Design review of the part built by this model. Coordinates are the model's own, in mm. A direction names the side the tool comes from. Coordinates: 2 decimals unless noted, no trailing zeros. Loops run counter-clockwise (first coordinate to the right, second up) from the corner with the lowest first, then second, coordinate; pieces in that order, holes last. Notation, with made-up numbers: M 21,36.25 L 67,36.25 A26 ccw 67,72.25 Z; hole C -4.5,45.25 d10. An arc over 180 degrees is marked long. One line per item, written item: value.
```python
from build123d import *

# Parameters (mm, degrees)
SKETCH1_R           = 5
BOSS_EXTRUDE1_DEPTH = 45
CHAMFER1_SIZE       = 1
CUT_EXTRUDE1_START  = -2
SKETCH2_R           = 6
SKETCH2_R_2         = 4
CUT_EXTRUDE1_DEPTH  = 1
CUT_EXTRUDE2_START  = -42
SKETCH2_2_R         = 6
SKETCH2_2_R_2       = 4
CUT_EXTRUDE2_DEPTH  = 1


with BuildPart() as part:
    # Sketch1 → Boss-Extrude1 (new body)
    with BuildSketch(Plane(origin=(0, 0, 0), x_dir=(1, 0, 0), z_dir=(0, 1, 0))):
        with Locations(Location((0, 0, 0), (0, 0, 90))):
            Circle(SKETCH1_R)
    extrude(amount=BOSS_EXTRUDE1_DEPTH)

    # Chamfer1
    chamfer1_edges = [part.edges().sort_by_distance(p)[0] for p in [
        (0, 0, 5),
        (0, 45, 5),
    ]]
    chamfer(chamfer1_edges, length=CHAMFER1_SIZE)

    # Sketch2 → Cut-Extrude1 (cut)
    with BuildSketch(Plane.XZ.offset(CUT_EXTRUDE1_START)):
        Circle(SKETCH2_R)
        with Locations(Location((0, 0, 0), (0, 0, 270))):
            Circle(SKETCH2_R_2, mode=Mode.SUBTRACT)
    extrude(amount=-CUT_EXTRUDE1_DEPTH, mode=Mode.SUBTRACT)

    # Sketch2_2 → Cut-Extrude2 (cut)
    with BuildSketch(Plane.XZ.offset(CUT_EXTRUDE2_START)):
        Circle(SKETCH2_2_R)
        with Locations(Location((0, 0, 0), (0, 0, 270))):
            Circle(SKETCH2_2_R_2, mode=Mode.SUBTRACT)
    extrude(amount=-CUT_EXTRUDE2_DEPTH, mode=Mode.SUBTRACT)


solid = part.part
```
(1) Tool access review of faces 4 (the cylindrical face through (-3.905, 2.493, 0.867)), 5 (the cylindrical face through (4.88, 1.49, 1.08)): name each direction out of +Z, -Z, +X, -X, +Y, -Y from which nothing blocks a thin tool from reaching the whole face with its end or side.
Reply:
face 4: none
face 5: +Y, -Y
(2) Mouldability with a two-part tool opening along Y and no side actions: class faces 1 (the flat face through (0, 45, 0)), 2 (the cylindrical face through (4.88, 43.49, 1.08)), 3 (the cylindrical face through (-3.905, 42.493, 0.867)) as released by +Y, released by -Y, zero draft, split by the parting line, or undercut.
Reply:
face 1: released by +Y
face 2: zero draft
face 3: undercut
(3) We need section A-A on y = 15. State the section outline as (x, z) points.
Reply:
outline: C 0,0 d10
(4) Insertion check: pin 1 (2 mm diameter, centred on x = 3, z = 3, fed in from -Y); pin 2 (5 mm diameter, centred on y = 35.5, z = 3.5, fed in from +X); pin 3 (1.5 mm diameter, centred on y = 4.5, z = -3.5, fed in from -X). Each pin has a flat end and moves straight along its axis. Give the tip position at first contact, or say it passes through.
Reply:
pin 1: stops at y = 0
pin 2: stops at x = 4.9
pin 3: stops at x = -4.18
(5) To check wall thickness, follow line 1 along Y through (x, z) = (4.75, 0.5); line 2 along Y through (x, z) = (0.25, -4.5); line 3 along X through (y, z) = (14.5, 0.25). State the ranges of each line that lie inside material, in increasing order. Write a range as [from, to].
Reply:
line 1: y = [0.78, 2], [3, 42], [43, 44.22]
line 2: y = [0.51, 2], [3, 42], [43, 44.49]
line 3: x = [-4.99, 4.99]
